Build history of the part. All positions in model axes, mm. Coordinates: 2 decimals unless noted, no trailing zeros. Order: outer loops, then holes, each group sorted by start corner. A loop starts at its lowest first (then second) coordinate and runs counter-clockwise, first axis right, second up. Notation, with made-up numbers: (-0.75, 63) - (45.25, 63) arc R16 ccw to (45.25, 85) - close; hole circle Ø8 at (31.25, -0.5). An arc over 180 degrees is marked (long way). Return JSON: item names as keys, results as strings.
from build123d import *

# Parameters (mm, degrees)
F0_W     = 50
F0_H     = 20
F0_R     = 3.25
F1_DEPTH = 25
F2_R     = 5
F3_DEPTH = 20


with BuildPart() as f1:
    # F0 (on Front) → F1 (new body)
    with BuildSketch(Plane.XZ):
        with Locations((25, 10)):
            Rectangle(F0_W, F0_H)
        with Locations((6, 10)):
            Circle(F0_R, mode=Mode.SUBTRACT)
        with Locations((44, 10)):
            Circle(F0_R, mode=Mode.SUBTRACT)
    extrude(amount=-F1_DEPTH)


with BuildPart() as f3:
    # F2 (on Top) → F3 (new body)
    with BuildSketch(Plane.XY):
        with Locations((25, 12.5)):
            Circle(F2_R)
    extrude(amount=F3_DEPTH)


with BuildPart() as f1_1:
    add(f1.part)

    # F4: cut F3
    add(f3.part, mode=Mode.SUBTRACT)


solid = f1_1.part
1. Cut at C-C on x = 6. Give the cut face in (y, z).
Check values:
{"outline": "(0, 0) - (25, 0) - (25, 6.75) - (0, 6.75) - close; (0, 13.25) - (25, 13.25) - (25, 20) - (0, 20) - close"}
2. Cut at B-B on y = 12.5. Give the cut face in (x, z), plus the area to 3 significant figures.
Check values:
{"outline": "(0, 0) - (20, 0) - (20, 20) - (0, 20) - close; (30, 0) - (50, 0) - (50, 20) - (30, 20) - close; hole circle Ø6.5 at (6, 10); hole circle Ø6.5 at (44, 10)", "area": "734 mm²"}
3. Drop a flat-ended pin along its axis: pin 1 (5 mm diameter, centred on x = 44, z = 10, fed in from +Y). Give the stop position or say it passes through.
Check values:
{"pin 1": "through"}
4. Probe L1, parallel to X at y = 7.25, z = 9.75; L2, parallel to X at y = 1.5, z = 11.5; L3, parallel to Y at x = 25, z = 9.25. List the from-to ranges inside material, lowest first.
Check values:
{"L1": "0 to 2.76, 9.24 to 40.76, 47.24 to 50", "L2": "0 to 3.12, 8.88 to 41.12, 46.88 to 50", "L3": "0 to 7.5, 17.5 to 25"}
5. Cut at D-D on z = 16.75. Give the cut face in (x, y), plus the area to 3 significant figures.
Check values:
{"outline": "(0, 0) - (50, 0) - (50, 25) - (0, 25) - close; hole circle Ø10 at (25, 12.5)", "area": "1,170 mm²"}
6. Mould opens along X. For faces 1 (the cylindrical face through (47.1, 12.32, 10.98)), 2 (the flat face through (25, 0, 10)), 3 (the flat face through (50, 12, 10)), 4 (the cylindrical face through (20.005, 12.72, 9.86)) say: pulls with the +X half, pulls with the -X half, needs draft (parallel to the pull), parting line crosses it, or undercut.
Check values:
{"face 1": "undercut", "face 2": "needs draft", "face 3": "pulls with the +X half", "face 4": "undercut"}
7. Cut at A-A on z = 10. Give the cut face in (x, y).
Check values:
{"outline": "(0, 0) - (2.75, 0) - (2.75, 25) - (0, 25) - close; (9.25, 0) - (40.75, 0) - (40.75, 25) - (9.25, 25) - close; (47.25, 0) - (50, 0) - (50, 25) - (47.25, 25) - close; hole circle Ø10 at (25, 12.5)"}
